Could you check a few things on this model? Use its own coordinates, in mm. Face numbers are marked on the shaded views. A direction names the side the tool comes from. Round coordinates to 2 decimals unless told otherwise and drop trailing zeros. Loops run counter-clockwise (first coordinate to the right, second up) from the corner with the lowest first, then second, coordinate; pieces in that order, holes last. Notation, with made-up numbers: M 67,-33 L 86,-33 A21 cw 86,-13 Z; hole C -15.75,68 d6. An arc over 180 degrees is marked long. One line per item, written item: value. Start each with the question number.
Q1. Please list where these lines run through material, in increasing order: line 1 along Z through (x, y) = (-39, 5); line 2 along X through (y, z) = (30.5, -27); line 3 along Y through (x, z) = (-29.5, 1.15).
Q2. Imagine slicing it at D-D (y = 17). Please give me the cut outline in (x, z).
Q3. Thinking about a two-plate mould opening in X: for the marked faces 3, 4, 5 and 6, which applies, released by +X, released by -X, zero draft, split by the parting line, or undercut?
Q4. Imagine slicing it at C-C (y = 32). Please give me the cut outline in (x, z).
Q5. Imagine slicing it at A-A (x = -29.5). Please give me the cut outline in (y, z).
Q6. Imagine slicing it at B-B (z = -16). Please give me the cut outline in (x, y).
Q7. Which directions (+Z, -Z, +X, -X, +Y, -Y) give clear straight access to the entire face, cutting with the end or side of a thin tool? Please do the marked faces 1 and 2.
Q8. I'm going to push flat-ended pins straight in: pin 1 Ø0.9 at (x, z) = (29.5, -2.5) entering from +Y; pin 2 Ø7.5 at (x, z) = (-34, -56) entering from +Y; pin 3 Ø6 at (x, y) = (-27, 12.5) entering from -Z; pin 4 Ø5.5 at (y, z) = (17, -16) entering from +X. Where does each tip first touch, or does it pass through?
from build123d import *

# Parameters (mm, degrees)
SKETCH_1_R          = 1.52
EXTRUDE_2_DEPTH     = 3
SKETCH_2_W          = 84.5
SKETCH_2_H          = 3
EXTRUDE_3_DEPTH     = 58
SKETCH_3_W          = 3
SKETCH_3_H          = 32
EXTRUDE_4_DEPTH     = 58
SKETCH_5_R          = 2.1
CUT_EXTRUDE_1_DEPTH = 58
EXTRUDE_9_DEPTH     = 5
CUT_EXTRUDE_4_DEPTH = 4
SKETCH_15_W         = 7
SKETCH_15_H         = 7
EXTRUDE_10_DEPTH    = 7
CUT_EXTRUDE_5_DEPTH = 5


with BuildPart() as part:
    # 草图1 → 凸台-拉伸2 (new body)
    with BuildSketch(Plane.XY):
        Polygon((0, 0), (42.25, 0), (42.25, 35), (0, 35), (-42.25, 35), (-42.25, 0), align=None)
        with Locations((-29.5, 17)):
            Circle(SKETCH_1_R, mode=Mode.SUBTRACT)
        with Locations((29.5, 17)):
            Circle(SKETCH_1_R, mode=Mode.SUBTRACT)
    extrude(amount=EXTRUDE_2_DEPTH)

    # 草图2 → 凸台-拉伸3 (add)
    with BuildSketch(Plane(origin=(0, 0, 0), x_dir=(-1, 0, 0), z_dir=(0, 0, -1))):
        with Locations((0, 1.5)):
            Rectangle(SKETCH_2_W, SKETCH_2_H)
    extrude(amount=EXTRUDE_3_DEPTH)

    # 草图3 → 凸台-拉伸4 (add)
    with BuildSketch(Plane(origin=(0, 0, 0), x_dir=(-1, 0, 0), z_dir=(0, 0, -1))):
        with Locations((40.75, 19)):
            Rectangle(SKETCH_3_W, SKETCH_3_H)
        with Locations((-40.75, 19)):
            Rectangle(SKETCH_3_W, SKETCH_3_H)
    extrude(amount=EXTRUDE_4_DEPTH)

    # 草图5 → 切除-拉伸1 (cut)
    with BuildSketch(Plane(origin=(42.25, 0, 0), x_dir=(0, 0, -1), z_dir=(1, 0, 0))):
        with Locations((16, 17)):
            Circle(SKETCH_5_R)
    extrude(amount=-CUT_EXTRUDE_1_DEPTH, mode=Mode.SUBTRACT)

    # 草图12 → 凸台-拉伸9 (add)
    with BuildSketch(Plane(origin=(0, 0, 0), x_dir=(-1, 0, 0), z_dir=(0, 0, -1))):
        Polygon((-35, 28), (-35, 35), (-24, 35), (-24, 28), (-29.5, 28), align=None)
        Polygon((29.5, 28), (24, 28), (24, 35), (35, 35), (35, 28), align=None)
    extrude(amount=EXTRUDE_9_DEPTH)

    # 草图14 → 切除-拉伸4 (cut)
    with BuildSketch(Plane(origin=(0, 35, 0), x_dir=(1, 0, 0), z_dir=(0, 1, 0))):
        with BuildLine():
            ThreePointArc((-28.01, 2.5), (-29.184567453, 3.956228797), (-30.856446051, 3.116566387))
            Line((-30.856446051, 3.116566387), (-28.143553949, 1.883433613))
            ThreePointArc((-28.143553949, 1.883433613), (-28.043771203, 2.184567453), (-28.01, 2.5))
        make_face()
        with BuildLine():
            Line((-28.143553949, 1.883433613), (-30.856446051, 3.116566387))
            ThreePointArc((-30.856446051, 3.116566387), (-30.116566387, 1.143553949), (-28.143553949, 1.883433613))
        make_face()
        with BuildLine():
            ThreePointArc((30.99, 2.5), (29.815432547, 3.956228797), (28.143553949, 3.116566387))
            Line((28.143553949, 3.116566387), (30.856446051, 1.883433613))
            ThreePointArc((30.856446051, 1.883433613), (30.956228797, 2.184567453), (30.99, 2.5))
        make_face()
        with BuildLine():
            Line((30.856446051, 1.883433613), (28.143553949, 3.116566387))
            ThreePointArc((28.143553949, 3.116566387), (28.883433613, 1.143553949), (30.856446051, 1.883433613))
        make_face()
    extrude(amount=-CUT_EXTRUDE_4_DEPTH, mode=Mode.SUBTRACT)

    # 草图15 → 凸台-拉伸10 (add)
    with BuildSketch(Plane(origin=(0, 3, 0), x_dir=(1, 0, 0), z_dir=(0, 1, 0))):
        with Locations((35.75, 54.5)):
            Rectangle(SKETCH_15_W, SKETCH_15_H)
        with Locations((-35.75, 54.5)):
            Rectangle(SKETCH_15_W, SKETCH_15_H)
    extrude(amount=EXTRUDE_10_DEPTH)

    # 草图16 → 切除-拉伸5 (cut)
    with BuildSketch(Plane(origin=(0, 0, -58), x_dir=(-1, 0, 0), z_dir=(0, 0, -1))):
        with BuildLine():
            ThreePointArc((-34.26, 6.5), (-35.179801686, 7.876580503), (-36.803589104, 7.553589104))
            Line((-36.803589104, 7.553589104), (-34.696410896, 5.446410896))
            ThreePointArc((-34.696410896, 5.446410896), (-34.373419497, 5.929801686), (-34.26, 6.5))
        make_face()
        with BuildLine():
            Line((-34.696410896, 5.446410896), (-36.803589104, 7.553589104))
            ThreePointArc((-36.803589104, 7.553589104), (-36.803589104, 5.446410896), (-34.696410896, 5.446410896))
        make_face()
        with BuildLine():
            ThreePointArc((36.803589104, 7.553589104), (34.696410896, 7.553589104), (34.696410896, 5.446410896))
            Line((34.696410896, 5.446410896), (36.803589104, 7.553589104))
        make_face()
        with BuildLine():
            Line((36.803589104, 7.553589104), (34.696410896, 5.446410896))
            ThreePointArc((34.696410896, 5.446410896), (36.320198314, 5.123419497), (37.24, 6.5))
            ThreePointArc((37.24, 6.5), (37.126580503, 7.070198314), (36.803589104, 7.553589104))
        make_face()
    extrude(amount=-CUT_EXTRUDE_5_DEPTH, mode=Mode.SUBTRACT)


solid = part.part
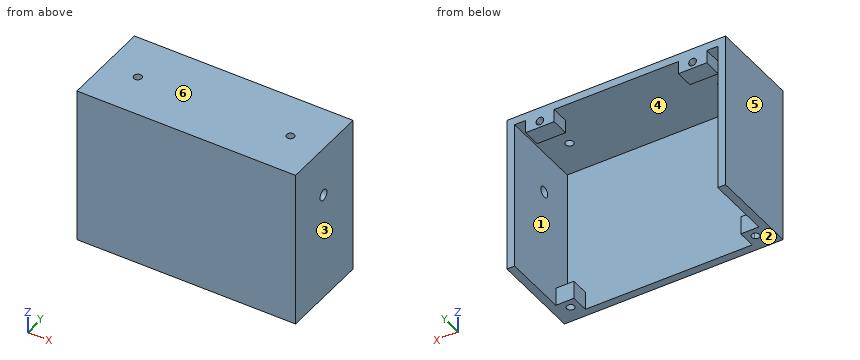
Report:
1. line 1: z = -58 to -51, 0 to 3
1. line 2: x = -42.25 to -39.25, 39.25 to 42.25
1. line 3: y = 0 to 15.48, 18.52 to 35
2. outline: M -42.25,-58 L -39.25,-58 L -39.25,0 L -31.02,0 L -31.02,3 L -42.25,3 Z; M -27.98,0 L 27.98,0 L 27.98,3 L -27.98,3 Z; M 31.02,0 L 39.25,0 L 39.25,-13.9 L 42.25,-13.9 L 42.25,3 L 31.02,3 Z; M 39.25,-58 L 42.25,-58 L 42.25,-18.1 L 39.25,-18.1 Z
3. face 3: released by +X
3. face 4: undercut
3. face 5: released by -X
3. face 6: zero draft
4. outline: M -42.25,-58 L -39.25,-58 L -39.25,0 L -35,0 L -35,-5 L -24,-5 L -24,0 L 24,0 L 24,-5 L 35,-5 L 35,0 L 39.25,0 L 39.25,-58 L 42.25,-58 L 42.25,3 L -42.25,3 Z; hole C -29.5,-2.5 d2.98; hole C 29.5,-2.5 d2.98
5. outline: M 0,-58 L 3,-58 L 3,0 L 15.48,0 L 15.48,3 L 0,3 Z; M 18.52,0 L 28,0 L 28,-5 L 35,-5 L 35,-3.99 L 31,-3.99 L 31,-1.01 L 35,-1.01 L 35,3 L 18.52,3 Z
6. outline: M -42.25,0 L 42.25,0 L 42.25,14.9 L 39.25,14.9 L 39.25,3 L -39.25,3 L -39.25,35 L -42.25,35 Z; M 39.25,19.1 L 42.25,19.1 L 42.25,35 L 39.25,35 Z
7. face 1: +Y
7. face 2: -Z, +X, -X, +Y, -Y
8. pin 1: stops at y = 31
8. pin 2: stops at y = 10
8. pin 3: stops at z = 0
8. pin 4: stops at x = 42.25
